Input: part model. Units: mm. Frame: model coordinates. A direction names the side the tool comes from. Give positions to 0.01 mm unless a question says otherwise; leave off trailing zeros. Order: outer loops, then holes, each group sorted by start corner. A loop starts at its lowest first (then second) coordinate and runs counter-clockwise, first axis right, second up. Notation, with made-up numbers: M 20,-35 L 40,-35 A36 cw 40,4 Z; hole C -4.5,34 d8. An arc over 180 degrees is marked long. Use a Markdown table: item, result.
from build123d import *

# Parameters (mm, degrees)
SKETCH_R        = 1.7
PAD_DEPTH       = 13
SKETCH001_W     = 42
SKETCH001_H     = 63.7
POCKET_DEPTH    = 10
SKETCH002_W     = 18.5
SKETCH002_H     = 7.5
POCKET001_DEPTH = 11
SKETCH003_R     = 3
POCKET002_DEPTH = 3.1


with BuildPart() as part:
    # Sketch → Pad (new body)
    with BuildSketch(Plane.XY):
        with BuildLine():
            Line((-5, -5), (-5, -77.7))
            ThreePointArc((-5, -77.7), (-3.535534, -81.235534), (0, -82.7))
            Line((0, -82.7), (51, -82.7))
            ThreePointArc((51, -82.7), (54.535534, -81.235534), (56, -77.7))
            Line((56, -77.7), (56, -5))
            ThreePointArc((56, -5), (54.535534, -1.464466), (51, 0))
            Line((51, 0), (0, 0))
            ThreePointArc((0, 0), (-3.535534, -1.464466), (-5, -5))
        make_face()
        with Locations((0, -5)):
            Circle(SKETCH_R, mode=Mode.SUBTRACT)
        with Locations((51, -5)):
            Circle(SKETCH_R, mode=Mode.SUBTRACT)
        with Locations((51, -77.7)):
            Circle(SKETCH_R, mode=Mode.SUBTRACT)
        with Locations((0, -77.7)):
            Circle(SKETCH_R, mode=Mode.SUBTRACT)
    extrude(amount=PAD_DEPTH)

    # Sketch001 (on Face14 of Pad) → Pocket (cut)
    with BuildSketch(Plane.XY.offset(13)):
        with Locations((25.5, -41.35)):
            Rectangle(SKETCH001_W, SKETCH001_H)
    extrude(amount=-POCKET_DEPTH, mode=Mode.SUBTRACT)

    # Sketch002 (on Face6 of Pocket) → Pocket001 (cut)
    with BuildSketch(Plane(origin=(0, 0, 0), x_dir=(-1, 0, 0), z_dir=(0, 1, 0))):
        with Locations((-26, 9.25)):
            Rectangle(SKETCH002_W, SKETCH002_H)
    extrude(amount=-POCKET001_DEPTH, mode=Mode.SUBTRACT)

    # Sketch003 (on Face4 of Pocket001) → Pocket002 (cut)
    with BuildSketch(Plane(origin=(0, 0, 0), x_dir=(1, 0, 0), z_dir=(0, 0, -1))):
        with Locations((0, 5)):
            Circle(SKETCH003_R)
        with Locations((51, 5)):
            Circle(SKETCH003_R)
        with Locations((51, 77.7)):
            Circle(SKETCH003_R)
        with Locations((0, 77.7)):
            Circle(SKETCH003_R)
    extrude(amount=-POCKET002_DEPTH, mode=Mode.SUBTRACT)


solid = part.part
1) First-contact query: pin 1 Ø5.5 at (x, y) = (0, -5) entering from +Z; pin 2 Ø4 at (x, y) = (51, -5) entering from -Z; pin 3 Ø4 at (y, z) = (-2.5, 8) entering from +X; pin 4 Ø1.5 at (x, y) = (13, -61.5) entering from +Z. Flat tips, straight axial feed; report the tip coordinate or a pass-through.
Response values:
| item | result |
|---|---|
| pin 1 | stops at z = 13 |
| pin 2 | stops at z = 3.1 |
| pin 3 | stops at x = 55.97 |
| pin 4 | stops at z = 3 |
2) Cut plane C-C on x = 43. Return loops of the section in (y, z), and give its area (3 significant figures).
Response values:
| item | result |
|---|---|
| outline | M -82.7,0 L 0,0 L 0,13 L -9.5,13 L -9.5,3 L -73.2,3 L -73.2,13 L -82.7,13 Z |
| area | 438 mm² |
3) Material intervals for line 1 (X direction, y = -77.7, z = 5.5); line 2 (X direction, y = -77.7, z = 1.5); line 3 (X direction, y = -5, z = 6), sorted ascending. Write a range as from..to.
Response values:
| item | result |
|---|---|
| line 1 | x = -5..-1.7, 1.7..49.3, 52.7..56 |
| line 2 | x = -5..-3, 3..48, 54..56 |
| line 3 | x = -5..-1.7, 1.7..16.75, 35.25..49.3, 52.7..56 |
4) Cut plane A-A on z = 8.5. Return loops of the section in (x, y), and give its area (3 significant figures).
Response values:
| item | result |
|---|---|
| outline | M -5,-77.7 A5 ccw 0,-82.7 L 51,-82.7 A5 ccw 56,-77.7 L 56,-5 A5 ccw 51,0 L 35.25,0 L 35.25,-9.5 L 46.5,-9.5 L 46.5,-73.2 L 4.5,-73.2 L 4.5,-9.5 L 16.75,-9.5 L 16.75,0 L 0,0 A5 ccw -5,-5 Z; hole C 0,-77.7 d3.4; hole C 0,-5 d3.4; hole C 51,-77.7 d3.4; hole C 51,-5 d3.4 |
| area | 2,140 mm² |
5) Cut plane B-B on y = -44.5. Return loops of the section in (x, z), and give its area (3 significant figures).
Response values:
| item | result |
|---|---|
| outline | M -5,0 L 56,0 L 56,13 L 46.5,13 L 46.5,3 L 4.5,3 L 4.5,13 L -5,13 Z |
| area | 373 mm² |
6) Mould query, pull axis Y, two halves, no side actions, for faces 5 (the face through (55, -2, 6)), 6 (the face through (2, -5, 3.1)), 7 (the face through (-5, -41, 6)). Classes: released by +Y, released by -Y, zero draft, split by the parting line, or undercut.
Response values:
| item | result |
|---|---|
| face 5 | released by +Y |
| face 6 | undercut |
| face 7 | zero draft |
7) Reachability of faces 1 (the face through (16.75, -5, 9)), 2 (the face through (46.5, -42, 8)), 3 (the face through (1, -76, 3.1)), 4 (the face through (49.3, -4.93, 7.98)) from +Z, -Z, +X, -X, +Y, -Y: full face, straight path, thin tool, end or side. Return the list, or none.
Response values:
| item | result |
|---|---|
| face 1 | +Z, +Y |
| face 2 | +Z |
| face 3 | -Z |
| face 4 | +Z, -Z |
